from build123d import *
from build123d import SkipClean  # not in build123d's __all__

# Parameters (mm, degrees)
F0_R          = 40.64
F1_DEPTH      = 10.16
F2_R          = 33.02
F3_DEPTH      = 5.08
F5_DEPTH      = 10.16
F6_R          = 6.35
F6_R_2        = 2.9972
F7_DEPTH      = 7.62
F7_DEPTH_BACK = 0.0127
F8_W          = 7.62
F8_H          = 2.54
F9_DEPTH      = 9.652


# Not quite as in the source:
# - after a boolean that leaves OpenCascade's solid faulty, fix() repairs it


with BuildPart() as f1:
    # F0 (on Top) → F1 (new body)
    with BuildSketch(Plane.XY):
        Circle(F0_R)
    extrude(amount=F1_DEPTH)

    # F2 (on face) → F3 (cut)
    with BuildSketch(Plane.XY.offset(10.16)):
        Circle(F2_R)
    extrude(amount=-F3_DEPTH, mode=Mode.SUBTRACT)

    # F4 (on face) → F5 (cut)
    with BuildSketch(Plane(origin=(0, 0, 0), x_dir=(1, 0, 0), z_dir=(0, 0, -1))):
        with BuildLine():
            Line((2.3139107243, -1.905), (-2.3139107243, -1.905))
            ThreePointArc((-2.3139107243, -1.905), (0, -2.9972), (2.3139107243, -1.905))
        make_face()
        with BuildLine():
            ThreePointArc((2.3139107243, -1.905), (2.8212108272, -1.0119176392), (2.9972, 0))
            ThreePointArc((2.9972, 0), (-1.0119176392, 2.8212108272), (-2.3139107243, -1.905))
            Line((-2.3139107243, -1.905), (2.3139107243, -1.905))
        make_face()
    extrude(amount=-F5_DEPTH, mode=Mode.SUBTRACT)

    # F6 (on face) → F7 (join, two sides)
    with BuildSketch(Plane.XY.offset(5.08)) as f7_sk:
        Circle(F6_R)
        Circle(F6_R_2, mode=Mode.SUBTRACT)
    with SkipClean():  # cleaning this boolean's faces spoils the solid; the shape is the same uncleaned
        extrude(amount=F7_DEPTH)
        extrude(f7_sk.sketch, amount=-F7_DEPTH_BACK)

    # F8 (on Top) → F9 (join)
    with BuildSketch(Plane.XY):
        with Locations((0, 3.175)):
            Rectangle(F8_W, F8_H)
    extrude(amount=F9_DEPTH)

    add(f1.part.fix(), mode=Mode.REPLACE)


solid = f1.part
Read the model definition and answer for the solid it produces. Units are mm, in the model's axes. A direction names the side the tool comes from. Give positions to 0.01 mm unless a question says otherwise; leave off trailing zeros. Loops run counter-clockwise (first coordinate to the right, second up) from the corner with the lowest first, then second, coordinate; pieces in that order, holes last. Notation, with made-up numbers: (46.5, 35) -> (88.5, 35) arc R25 cw to (88.5, 52) -> close; hole circle Ø9 at (-21, 48.25). An arc over 180 degrees is marked (long way). Use a Markdown table: item, result.
Q1. Section D-D, the plane y = 12.5 is taken. Determine the outline of the cut face in (x, z).
Solved:
| item | result |
|---|---|
| outline | (-38.67, 0) -> (38.67, 0) -> (38.67, 10.16) -> (30.56, 10.16) -> (30.56, 5.08) -> (-30.56, 5.08) -> (-30.56, 10.16) -> (-38.67, 10.16) -> close |
Q2. Determine the mould class of faces 3 (the face through (8, 1, 0)), 4 (the face through (-5.291, 40.294, 5.009)), 5 (the face through (0, 1.905, 5)) for opening direction Y: pulls with the +Y half, pulls with the -Y half, needs draft (parallel to the pull), parting line crosses it, or undercut.
Solved:
| item | result |
|---|---|
| face 3 | needs draft |
| face 4 | parting line crosses it |
| face 5 | undercut |
Q3. Each of these flat-tipped pins is pushed along its axis until it touches: pin 1 (2.5 mm diameter, centred on x = -0.5, z = 6.5, fed in from -Y); pin 2 (2 mm diameter, centred on y = 2.5, z = 10, fed in from +X); pin 3 (1 mm diameter, centred on x = 31, z = 8, fed in from +Y). Where does it stop, or does it pass through?
Solved:
| item | result |
|---|---|
| pin 1 | stops at y = -40.64 |
| pin 2 | stops at x = 40.61 |
| pin 3 | stops at y = 26.86 |
Q4. A tool of negligible diameter and unlimited length cuts with its end or side. For faces 1 (the face through (31.5, 9.9, 7.7)), 2 (the face through (3, -1, 12.7)), from which of +Z, -Z, +X, -X, +Y, -Y can it reach the whole face along a straight path? Write none if from no direction.
Solved:
| item | result |
|---|---|
| face 1 | +Z |
| face 2 | +Z, +X, -X, +Y, -Y |
Q5. Section C-C, the plane x = 21 is taken. Determine the outline of the cut face in (y, z), then the cut area to 3 significant figures.
Solved:
| item | result |
|---|---|
| outline | (-34.79, 0) -> (34.79, 0) -> (34.79, 10.16) -> (25.48, 10.16) -> (25.48, 5.08) -> (-25.48, 5.08) -> (-25.48, 10.16) -> (-34.79, 10.16) -> close |
| area | 448 mm^2 |
Q6. Section A-A, the plane x = 0 is taken. Determine the outline of the cut face in (y, z) (3 decimals), then the cut area to 3 significant figures.
Solved:
| item | result |
|---|---|
| outline | (-40.64, 0) -> (-2.997, 0) -> (-2.997, 12.7) -> (-6.35, 12.7) -> (-6.35, 5.08) -> (-33.02, 5.08) -> (-33.02, 10.16) -> (-40.64, 10.16) -> close; (1.905, 0) -> (40.64, 0) -> (40.64, 10.16) -> (33.02, 10.16) -> (33.02, 5.08) -> (6.35, 5.08) -> (6.35, 12.7) -> (2.997, 12.7) -> (2.997, 9.652) -> (1.905, 9.652) -> close |
| area | 522 mm^2 |
Q7. Section B-B, the plane z = 4 is taken. Determine the outline of the cut face in (x, y) (3 decimals).
Solved:
| item | result |
|---|---|
| outline | circle Ø81.28 at (0, 0); hole (-2.314, 1.905) arc R2.997 ccw (long way) to (2.314, 1.905) -> close |
Q8. Find the intervals of material crossed by line 1 along Y through (x, z) = (0, 8.6) (3 decimals); line 2 along Y through (x, z) = (0, 10); line 3 along Y through (x, z) = (0, 4.5) (3 decimals), in increasing order.
Solved:
| item | result |
|---|---|
| line 1 | y = -40.64 to -33.02, -6.35 to -2.997, 1.905 to 6.35, 33.02 to 40.64 |
| line 2 | y = -40.64 to -33.02, -6.35 to -3, 3 to 6.35, 33.02 to 40.64 |
| line 3 | y = -40.64 to -2.997, 1.905 to 40.64 |
